```python
from build123d import *

# Parameters (mm, degrees)
SKETCH1_R            = 9.525
EXTRUDE1_DEPTH       = 19.05
CHAMFER1_SIZE        = 0.4064
TRUNCATED_DEPTH      = 20.05
TRUNCATED_DEPTH_BACK = 20.05
SKETCH6_R            = 2.38125
BLIND_HOLES_DEPTH    = 4.7625


with BuildPart() as part:
    # Sketch1 → Extrude1 (new body, symmetric)
    with BuildSketch(Plane.XY):
        Circle(SKETCH1_R)
    extrude(amount=EXTRUDE1_DEPTH, both=True)

    # Chamfer1
    chamfer1_edges = [part.edges().sort_by_distance(p)[0] for p in [
        (-9.525, 0, -19.05),
        (-9.525, 0, 19.05),
    ]]
    chamfer(chamfer1_edges, length=CHAMFER1_SIZE)

    # Sketch2 → Truncated (cut, two sides)
    with BuildSketch(Plane.XY) as truncated_sk:
        with BuildLine():
            Line((-8.980256121, -3.175), (8.980256121, -3.175))
            ThreePointArc((8.980256121, -3.175), (0, -9.525), (-8.980256121, -3.175))
        make_face()
    extrude(amount=TRUNCATED_DEPTH, mode=Mode.SUBTRACT)
    extrude(truncated_sk.sketch, amount=-TRUNCATED_DEPTH_BACK, mode=Mode.SUBTRACT)

    # Sketch6 → Blind Holes (cut)
    with BuildSketch(Plane(origin=(0, -3.175, 0), x_dir=(-1, 0, 0), z_dir=(0, 1, 0))):
        with Locations(Location((0, 12.7, 0), (0, 0, 90))):  # turned: the seam where the file's is
            Circle(SKETCH6_R)
        with Locations(Location((0, -12.7, 0), (0, 0, 90))):  # turned: the seam where the file's is
            Circle(SKETCH6_R)
    extrude(amount=BLIND_HOLES_DEPTH, mode=Mode.SUBTRACT)


solid = part.part
```
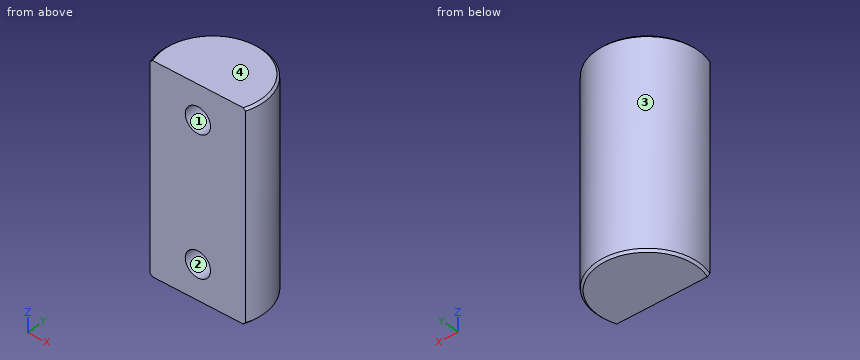
Part model, mm, in its own coordinate system. Face numbers are marked on the shaded views. Coordinates: 2 decimals unless noted, no trailing zeros. Write each loop counter-clockwise with the first axis right and the second up, starting at its lowest first coordinate (ties: lowest second). Pieces come first, ordered by that corner, then holes.
Item 1: Pin check, flat tips, straight feed: pin 1 (1.4 mm diameter, centred on x = 0, z = -12, fed in from -Y); pin 2 (5 mm diameter, centred on x = -0.5, z = 12.5, fed in from -Y) (3 decimals); pin 3 (6 mm diameter, centred on y = 7.5, z = -1.5, fed in from -X) (3 decimals); pin 4 (2 mm diameter, centred on y = 2.5, z = -12, fed in from -X). Stop position of each tip, or through.
Item 2: Mould opens along Z. For the marked faces 1, 2, 3 and 4 say: released by +Z, released by -Z, zero draft, split by the parting line, or undercut.
Item 3: Probe line 1 (X direction, y = -0.25, z = -12.7); line 2 (X direction, y = -1.95, z = 12.7); line 3 (Y direction, x = -2.75, z = 16) (3 decimals). List the from-to ranges inside material, lowest first.
Item 4: Slice it at A-A (y = 0). Count the separate pieces of the cut face and the enclosed holes in it, and give its area (3 significant figures).
Item 5: Slice it at D-D (z = -0.5). Write the cut outline in (x, y) (3 decimals).
Results found:
1. pin 1: stops at y = 1.59
1. pin 2: stops at y = -3.175
1. pin 3: stops at x = -8.395
1. pin 4: stops at x = -9.41
2. face 1: undercut
2. face 2: undercut
2. face 3: zero draft
2. face 4: released by +Z
3. line 1: x = -9.52 to -2.38, 2.38 to 9.52
3. line 2: x = -9.32 to -2.38, 2.38 to 9.32
3. line 3: y = -3.175 to 9.119
4. separate pieces: 1
4. enclosed holes: 2
4. area: 690 mm2
5. outline: (-8.98, -3.175) - (8.98, -3.175) arc R9.525 ccw (long way) to start
